from build123d import *


with BuildPart() as part:
    # Эскиз1 → Повернуть1 (revolve)
    with BuildSketch(Plane(origin=(0, 0, 0), x_dir=(1, 0, 0), z_dir=(0, 1, 0))):
        with BuildLine():
            Line((5, 0), (5, 4))
            Line((5, 4), (4.25, 7.698728048))
            ThreePointArc((4.25, 7.698728048), (3.902903442, 8.27418604), (3.269945327, 8.5))
            Line((3.269945327, 8.5), (1.5, 8.5))
            Line((1.5, 8.5), (1.5, 7.1))
            Line((1.5, 7.1), (3.75, 7.1))
            Line((3.75, 7.1), (3.75, 0))
            Line((3.75, 0), (5, 0))
        make_face()
    revolve(axis=Axis((0, 0, 0), (0, 0, -1)))


solid = part.part
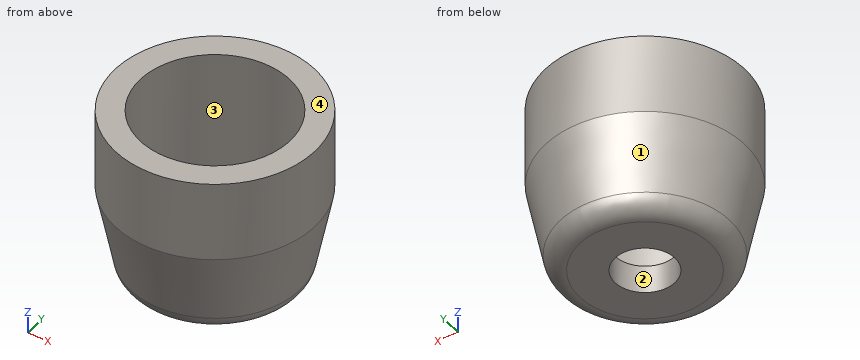
Model file for the job. Use its own axes, mm. Face numbers are marked on the shaded views. Give positions to 0.01 mm unless a question says otherwise; leave off trailing zeros. Write each loop counter-clockwise with the first axis right and the second up, starting at its lowest first coordinate (ties: lowest second). Pieces come first, ordered by that corner, then holes. Notation, with made-up numbers: (-39, 47) - (-30, 47) arc R23 ccw to (-30, 86) - close; hole circle Ø3 at (-17.75, 79.25). An arc over 180 degrees is marked (long way). Answer as CSV lines item,"result".
1. Drill centre lines: L1, parallel to Y at x = 0, z = -3.25; L2, parallel to X at y = 0, z = -5.5. Where is each one in solid material? Low to high. Write a range as [from, to].
Responses:
L1,"y = [-5, -3.75], [3.75, 5]"
L2,"x = [-4.7, -3.75], [3.75, 4.7]"
2. Band-saw the part on D-D (z = -6.75). Write the cut outline in (x, y).
Responses:
outline,"circle Ø8.88 at (0, 0); hole circle Ø7.5 at (0, 0)"
3. Pin check, flat tips, straight feed: pin 1 (2 mm diameter, centred on x = 0.5, y = 3, fed in from +Z); pin 2 (6 mm diameter, centred on x = 0, y = 0, fed in from +Z). Stop position of each tip, or through.
Responses:
pin 1,"stops at z = 0"
pin 2,"stops at z = -7.1"
4. Band-saw the part on A-A (y = 0). Write the cut outline in (x, z).
Responses:
outline,"(-5, -4) - (-4.25, -7.7) arc R1 ccw to (-3.27, -8.5) - (-1.5, -8.5) - (-1.5, -7.1) - (-3.75, -7.1) - (-3.75, 0) - (-5, 0) - close; (1.5, -8.5) - (3.27, -8.5) arc R1 ccw to (4.25, -7.7) - (5, -4) - (5, 0) - (3.75, 0) - (3.75, -7.1) - (1.5, -7.1) - close"
5. Band-saw the part on C-C (z = -3). Write the cut outline in (x, y).
Responses:
outline,"circle Ø10 at (0, 0); hole circle Ø7.5 at (0, 0)"
6. Two-plate mould, pull along Y, no slides. Class the marked faces 1, 2, 3 and 4: +Y half, -Y half, draft (parallel to the pull), parting line (faces both ways), or undercut.
Responses:
face 1,"parting line"
face 2,"undercut"
face 3,"undercut"
face 4,"draft"
